Input: part model. Units: mm. Frame: model coordinates. Face numbers are marked on the shaded views. A direction names the side the tool comes from. Round coordinates to 2 decimals unless told otherwise and drop trailing zeros. Write each loop counter-clockwise with the first axis right and the second up, starting at its lowest first coordinate (ties: lowest second). Pieces come first, ordered by that corner, then holes. Notation, with made-up numbers: M 34.5,8.25 L 38.5,8.25 A31 ccw 38.5,47.25 Z; hole C -35.75,82.25 d10. An arc over 180 degrees is marked long. Write each question's results on one line, items separated by ' | '. Start each with the question number.
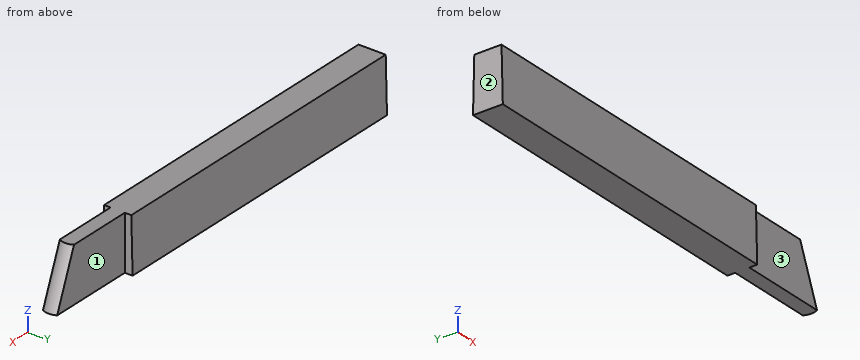
Autodesk Inventor part; units mm, degrees
ref_plane "Work Plane1" through (0, 0, 50.8) normal (0, 0, 1) x (1, 0, 0)
ref_plane "YZ Plane" through (0, 0, 0) normal (1, 0, 0) x (0, 1, 0)
ref_plane "XZ Plane" through (0, 0, 0) normal (0, 1, 0) x (-1, 0, 0)
sketch "Sketch2" plane through (0, 0, 0) normal (0, 0, 1) x (1, 0, 0)
  line L0 (0, 0) -> (25.4, 0)
  line L1 (25.4, 0) -> (25.4, 5.588)
  line L2 (25.4, 5.588) -> (0, 5.588)
  line L3 (0, 5.588) -> (0, 0)
  arc A0 (25.4, 0) -> (25.4, 5.588) centre (25.4, 2.794) ccw
  dimension "d0" = 25.4
  dimension "d1" = 5.588
ref_plane "Work Plane1" through (0, 0, 50.8) normal (0, 0, 1) x (1, 0, 0)
sketch "Sketch3" plane through (0, 0, 50.8) normal (0, 0, 1) x (1, 0, 0)
  line L0 (0, 1.2065) -> (6.35, 1.2065)
  line L1 (6.35, 1.2065) -> (6.35, 4.3815)
  line L2 (6.35, 4.3815) -> (0, 4.3815)
  line L3 (0, 4.3815) -> (0, 1.2065)
  arc A0 (6.35, 1.2065) -> (6.35, 4.3815) centre (6.35, 2.794) ccw
  point P0 (0, 0)
  dimension "d3" = 6.35
  dimension "d4" = 3.175
  dimension "d5" = 1.2065
loft "Loft1" add profiles "Sketch2", "Sketch3"
sketch "Sketch4" plane through (0, 0, 0) normal (-1, 0, 0) x (0, 0, 1)
  line L0 (0, 5.588) -> (0, 0)
  line L1 (0, 0) -> (50.8, 1.2065)
  line L2 (50.8, 4.3815) -> (50.8, 1.2065)
  line L3 (0, 5.588) -> (50.8, 4.3815)
  line L4 (0, 5.588) -> (50.8, 4.3815)
  line L5 (44.45, 4.5323) -> (44.45, 1.0557)
  line L6 (50.8, 1.2065) -> (0, 0)
  dimension "d10" = 6.35
extrude "Extrusion1" add sketch "Sketch4" along normal blind 38.608 contours L3 L2 L1 L5
sketch "Sketch5" plane through (25.4, 5.588, 0) normal (0, 0, -1) x (-1, 0, 0)
  line L0 (25.4, 0) -> (25.4, -5.588)
  line L1 (0, 0) -> (25.4, 0)
  arc A0 (0, 0) -> (0, -5.588) centre (0, -2.794) ccw
  line L2 (25.4, -5.588) -> (0, -5.588)
  line L3 (25.4, 0) -> (25.4, -5.588)
  line L4 (25.4, 0) -> (36.1487, 0)
  line L5 (36.1487, 0) -> (36.1487, -5.5776)
  line L6 (36.1487, -5.5776) -> (25.4, -5.5776)
  line L7 (25.4, -5.5776) -> (25.4, 0)
  line L8 (-3.175, -0.1076) -> (-3.175, -7.007)
  line L9 (25.4, -5.588) -> (0, -5.588)
revolve "Revolution1" add sketch "Sketch5" angle 15 about axis through (28.575, 5.4804, 0) along (0, -1, 0)
sketch "Sketch7" plane through (-10.7487, 5.588, 0) normal (0, 1, 0) x (1, 0, 0)
  line L0 (0, 0) -> (10.7487, 0)
  line L1 (36.1487, 0) -> (10.7487, 0)
  arc A0 (36.2569, 0.8218) -> (36.1487, 0) centre (39.3237, 0) ccw
  line L2 (1.3399, 10.1777) -> (36.2569, 0.8218)
  arc A1 (1.3399, 10.1777) -> (0, 0) centre (39.3237, 0) ccw
  line L3 (10.7487, 0) -> (10.7487, -44.45)
  line L4 (10.7487, 0) -> (-2.0556, 0)
  line L5 (-2.0556, 0) -> (-2.0556, 10.6947)
  line L6 (-2.0556, 10.6947) -> (10.7487, 10.6947)
  line L7 (10.7487, 10.6947) -> (10.7487, 0)
extrude "Extrusion2" cut sketch "Sketch7" against normal blind 38.1 contours A1 L2 L7 L0 | L4 L5 L6 L7 L2 A1
sketch "Sketch8" plane through (0, 0.0104, -7.6566) normal (0.258819, 0, -0.9659258) x (-0.9659258, 0, -0.258819)
  line L0 (-29.583, 2.7836) -> (-24.8205, 2.7836)
  line L1 (-24.8205, 2.7836) -> (-8.9455, 2.7836)
  circle A0 centre (-24.8205, 2.7836) radius 1.27
  circle A1 centre (-8.9455, 2.7836) radius 1.27
  line L2 (-26.408, -0.0104) -> (0, -0.0104)
  point P0 (-1.9817, -0.0104)
  point P1 (0, 0)
  dimension "d17" = 4.7625
  dimension "d18" = 15.875
  dimension "d19" = 2.54
  dimension "d20" = 2.54
  dimension "d23" = 2.794
extrude "Extrusion4" cut sketch "Sketch8" against normal blind 12.7
sketch "Sketch9" plane through (0, 1.0557, 44.45) normal (-1, 0, 0) x (0, 0, 1)
  line L0 (6.35, 0.1508) -> (6.35, 3.3258)
  line L1 (6.35, 3.3258) -> (0, 3.4766)
  line L2 (0, 3.4766) -> (0, 0)
  line L3 (0, 0) -> (6.35, 0.1508)
  line L4 (6.35, 3.3258) -> (6.35, 0.1508)
  line L5 (6.35, 2.5638) -> (0, 2.5638)
  line L6 (0, 3.4766) -> (0, 0)
  line L7 (6.35, 0.9128) -> (0, 0.9128)
  line L8 (6.35, 2.5638) -> (6.35, 4.769)
  line L9 (6.35, 4.769) -> (-56.0869, 8.5681)
  line L10 (-56.0869, 8.5681) -> (-57.3905, -12.8563)
  line L11 (-57.3905, -12.8563) -> (6.35, -0.7759)
  line L12 (6.35, -0.7759) -> (6.35, 0.9128)
  line L13 (0, 0.9128) -> (0, 0) construction
  line L14 (0, 2.5638) -> (0, 3.4766) construction
  line L15 (0, 2.5638) -> (0, 0.9128)
  point P0 (-44.45, -1.0557)
  dimension "d26" = 1.651
extrude "Extrusion5" cut sketch "Sketch9" against normal through all contours L3 L2 L7 L0 | L12 L11 L10 L9 L8 L1 L2 L3 | L5 L2 L1 L0
properties part number "DivePlanesStabilizingFins_Print2"
1. Cut plane A-A on x = -8. Output: boundary loops of the cut face in (y, z), and give its area (3 significant figures).
2. Contact query for flat-ended pins moving along their axis: P1, Ø3, axis at x = 5, z = 47.5, coming from the +Y side; P2, Ø3, axis at x = -8.5, z = 50, coming from the +Y side; P3, Ø1, axis at y = 4, z = 47, coming from the +X side. Output: stop coordinate, or through.
3. Access query for the marked faces 1, 2 and 3. Directions: +Z, -Z, +X, -X, +Y, -Y. A direction counts if a zero-diameter tool reaches every point of the face in a straight line with its end or side. Return the directions, or none.
4. Cut plane B-B on x = 2.5. Output: boundary loops of the cut face in (y, z).
5. Line query: L1, parallel to X at y = 1.5, z = 47.25; L2, parallel to Y at x = 3.5, z = 47; L3, parallel to X at y = 2.2, z = 47.5. Output: solid intervals per line, ascending. Write a range as from..to.
Answers follow:
1) outline: M 1.06,44.45 L 4.53,44.45 L 4.38,50.8 L 1.21,50.8 Z | area: 21.1 mm2
2) P1: stops at y = 3.62 | P2: stops at y = 4.44 | P3: stops at x = 9.37
3) face 1: +Z, -Z, +X, +Y | face 2: +Z, -Z, -X, +Y, -Y | face 3: +Z, -Z, +X, -Y
4) outline: M 1.97,44.45 L 3.62,44.45 L 3.62,50.8 L 1.97,50.8 Z
5) L1: x = -38.61..0 | L2: y = 1.97..3.62 | L3: x = -38.61..9.14
